```python
from build123d import *

# Parameters (mm, degrees)
SKETCH1_W               = 27.6
SKETCH1_H               = 30
BASE_FLANGE1_DEPTH      = 2
EDGE_FLANGE1_DEPTH      = 30
EDGE_FLANGE1_BEND_DEPTH = 30


# Sheet-metal steps are written as plain solids
with BuildPart() as part:
    # Sketch1 → Base-Flange1 (new body)
    with BuildSketch(Plane(origin=(0, 0, 0), x_dir=(1, 0, 0), z_dir=(0, 1, 0))):
        Rectangle(SKETCH1_W, SKETCH1_H)
    extrude(amount=-BASE_FLANGE1_DEPTH)

    # Edge-Flange1 section (across the edge) → Edge-Flange1 (add)
    with BuildSketch(Plane(origin=(15, 0, 15), x_dir=(-1, 0, 0), z_dir=(0, 0, -1))):
        with BuildLine():
            Line((-2, 1.2), (-2, 28))
            Line((-2, 28), (0, 28))
            Line((0, 28), (0, 1.2))
            ThreePointArc((0, 1.2), (0.351471863, 0.351471863), (1.2, 0))
            Line((1.2, 0), (1.2, -2))
            ThreePointArc((1.2, -2), (-1.0627417, -1.0627417), (-2, 1.2))
        make_face()
    extrude(amount=EDGE_FLANGE1_DEPTH)

    # Edge-Flange1 section 2 (across the edge) → Edge-Flange1 bend (add)
    with BuildSketch(Plane(origin=(-15, 0, -15), x_dir=(1, 0, 0), z_dir=(0, 0, 1))):
        with BuildLine():
            Line((-2, 1.2), (-2, 28))
            Line((-2, 28), (0, 28))
            Line((0, 28), (0, 1.2))
            ThreePointArc((0, 1.2), (0.351471863, 0.351471863), (1.2, 0))
            Line((1.2, 0), (1.2, -2))
            ThreePointArc((1.2, -2), (-1.0627417, -1.0627417), (-2, 1.2))
        make_face()
    extrude(amount=EDGE_FLANGE1_BEND_DEPTH)


solid = part.part
```
Verification items for the finished model (mm, model axes). A direction names the side the tool comes from. Coordinates: 2 decimals unless noted, no trailing zeros. Loops run counter-clockwise (first coordinate to the right, second up) from the corner with the lowest first, then second, coordinate; pieces in that order, holes last. Notation, with made-up numbers: (78, 29) -> (82, 29) arc R7 cw to (82, 36) -> close; hole circle Ø1 at (58.5, -7.5). An arc over 180 degrees is marked (long way). Answer in a Markdown table with one row per item.
1) Section check A-A (y = 18.75). Record the cut outline in (x, z), and give its area (3 significant figures).
The answers:
| item | result |
|---|---|
| outline | (-17, -15) -> (-15, -15) -> (-15, 15) -> (-17, 15) -> close; (15, -15) -> (17, -15) -> (17, 15) -> (15, 15) -> close |
| area | 120 mm2 |
2) Access from +Z, -Z, +X, -X, +Y, -Y to the whole of each face (thin tool, end or side, straight path). Record for faces 4 (the face through (15, 15, 0)), 5 (the face through (16, 28, 0)).
The answers:
| item | result |
|---|---|
| face 4 | +Z, -Z, +Y |
| face 5 | +Z, -Z, +X, -X, +Y |
3) Depth check by flat-ended pin: P1, Ø1.5, axis at x = -11.5, z = 4, coming from the +Y side. Enter the tip coordinate at first touch or a pass-through.
The answers:
| item | result |
|---|---|
| P1 | stops at y = 0 |
4) Scan lines: line 1 along X through (y, z) = (26.25, -3); line 2 along Y through (x, z) = (-11.5, 4.75). Record each from-to range of solid material in increasing order. Write a range as from..to.
The answers:
| item | result |
|---|---|
| line 1 | x = -17..-15, 15..17 |
| line 2 | y = -2..0 |
5) Draft check along X on faces 1 (the face through (16.038, -1.087, 0.21)), 2 (the face through (-16.038, -1.087, -0.21)), 3 (the face through (-14.658, 0.361, -0.21)). Enter one of: released by +X, released by -X, zero draft, split by the parting line, or undercut.
The answers:
| item | result |
|---|---|
| face 1 | released by +X |
| face 2 | released by -X |
| face 3 | undercut |
6) Section check C-C (x = 6). Record the cut outline in (y, z), and give its area (3 significant figures).
The answers:
| item | result |
|---|---|
| outline | (-2, -15) -> (0, -15) -> (0, 15) -> (-2, 15) -> close |
| area | 60.0 mm2 |
7) Section check B-B (z = 9). Record the cut outline in (x, y), and give its area (3 significant figures).
The answers:
| item | result |
|---|---|
| outline | (-17, 1.2) arc R3.2 ccw to (-13.8, -2) -> (13.8, -2) arc R3.2 ccw to (17, 1.2) -> (17, 28) -> (15, 28) -> (15, 1.2) arc R1.2 cw to (13.8, 0) -> (-13.8, 0) arc R1.2 cw to (-15, 1.2) -> (-15, 28) -> (-17, 28) -> close |
| area | 176 mm2 |
